```python
from build123d import *

# Parameters (mm, degrees)
F1_DEPTH = 310


with BuildPart() as f1:
    # F0 (on Front) → F1 (new body)
    with BuildSketch(Plane.XZ):
        with BuildLine():
            Line((2.17, 19.1), (0, 19.1))
            Line((0, 19.1), (0, 0))
            Line((0, 0), (19.1, 0))
            Line((19.1, 0), (19.1, 2.17))
            ThreePointArc((19.1, 2.17), (18.807107, 2.877107), (18.1, 3.17))
            Line((18.1, 3.17), (4.17, 3.17))
            ThreePointArc((4.17, 3.17), (3.462893, 3.462893), (3.17, 4.17))
            Line((3.17, 4.17), (3.17, 18.1))
            ThreePointArc((3.17, 18.1), (2.877107, 18.807107), (2.17, 19.1))
        make_face()
    extrude(amount=F1_DEPTH)


solid = f1.part
```
Could you check a few things on this model? Use its own coordinates, in mm. A direction names the side the tool comes from. Round coordinates to 2 decimals unless told otherwise and drop trailing zeros. Loops run counter-clockwise (first coordinate to the right, second up) from the corner with the lowest first, then second, coordinate; pieces in that order, holes last.
Q1. Please list where these lines run through material, in increasing order: L1, parallel to Z at x = 17.75, y = -277; L2, parallel to X at y = -218, z = 18.25; L3, parallel to Z at x = 3, y = -180.5.
Q2. On a 3-axis mill with a long thin cutter (end or side, diameter ignored), from which of +Z, -Z, +X, -X, +Y, -Y can I reach the whole of each face in a straight line? I mean faces 1 (the flat face through (3, -310, 6)), 2 (the flat face through (3.17, -153, 11)). Say none if no direction works.
Q3. For P1, Ø10, axis at y = -167, z = 7, coming from the -X side; P2, Ø3, axis at y = -85.5, z = 12.5, coming from the +X side; P3, Ø7, axis at x = 12.5, y = -201, coming from the +Z side, each with a flat end and sliding along its axis, tell me the tip position at first contact or that it passes through.
Q4. I want a section at C-C (z = 15.5). Write out the boundary of the cut face in (x, y), and give its area (3 significant figures).
Q5. I want a section at B-B (x = 11). Write out the boundary of the cut face in (y, z), and give its area (3 significant figures).
Q6. I want a section at A-A (y = -31.5). Write out the boundary of the cut face in (x, z).
Answer below:
1. L1: z = 0 to 3.17
1. L2: x = 0 to 3.16
1. L3: z = 0 to 18.66
2. face 1: +Z, -Z, +X, -X, -Y
2. face 2: +Z, +X, +Y, -Y
3. P1: stops at x = 0
3. P2: stops at x = 3.17
3. P3: stops at z = 3.17
4. outline: (0, -310) - (3.17, -310) - (3.17, 0) - (0, 0) - close
4. area: 983 mm2
5. outline: (-310, 0) - (0, 0) - (0, 3.17) - (-310, 3.17) - close
5. area: 983 mm2
6. outline: (0, 0) - (19.1, 0) - (19.1, 2.17) arc R1 ccw to (18.1, 3.17) - (4.17, 3.17) arc R1 cw to (3.17, 4.17) - (3.17, 18.1) arc R1 ccw to (2.17, 19.1) - (0, 19.1) - close
